Read the model definition and answer for the solid it produces. Units are mm, in the model's axes. A direction names the side the tool comes from. Give positions to 0.01 mm unless a question says otherwise; leave off trailing zeros. Write each loop counter-clockwise with the first axis right and the second up, starting at its lowest first coordinate (ties: lowest second). Pieces come first, ordered by that corner, then holes. Notation, with made-up numbers: (48, 84.5) - (75, 84.5) arc R15 ccw to (75, 101.5) - close; hole circle Ø4 at (61.25, 47). An arc over 180 degrees is marked (long way). Answer as CSV lines item,"result".
```python
from build123d import *

# Parameters (mm, degrees)
SKETCH2_R          = 2
CUT_EXTRUDE1_DEPTH = 10


with BuildPart() as part:
    # Sketch1 → Revolve1 (revolve)
    with BuildSketch(Plane.XY, mode=Mode.PRIVATE) as revolve1_sk:
        Polygon((0, 0), (132, 0), (132, 4), (114, 4), (114, 6), (112, 6), (112, 13), (110, 13), (110, 21), (0, 21), align=None)
    revolve(revolve1_sk.sketch.rotate(Axis((0, 0, 0), (1, 0, 0)), 180), axis=Axis((0, 0, 0), (1, 0, 0)))

    # Sketch2 → Cut-Extrude1 (cut)
    with BuildSketch(Plane(origin=(110, 0, 0), x_dir=(0, 0, -1), z_dir=(1, 0, 0))):
        with Locations(Location((0, 17.365813997, 0), (0, 0, 90))):
            Circle(SKETCH2_R)
        with Locations(Location((17.365813997, 0, 0), (0, 0, 90))):
            Circle(SKETCH2_R)
        with Locations(Location((0, -17.365813997, 0), (0, 0, 90))):
            Circle(SKETCH2_R)
        with Locations(Location((-17.365813997, 0, 0), (0, 0, 90))):
            Circle(SKETCH2_R)
    extrude(amount=-CUT_EXTRUDE1_DEPTH, mode=Mode.SUBTRACT)


solid = part.part
```
(1) Each of these flat-tipped pins is pushed along its axis until it touches: P1, Ø3, axis at x = 18, z = -11, coming from the +Y side; P2, Ø3, axis at y = 8, z = 11, coming from the +X side; P3, Ø1, axis at x = 61.5, y = 10, coming from the -Z side. Where does it stop, or does it pass through?
Worked out:
P1,"stops at y = 18.73"
P2,"stops at x = 112"
P3,"stops at z = -18.73"
(2) A cutting plane is placed at C-C (x = 30). Write down the section's boundary in (y, z), and give its area (3 significant figures).
Worked out:
outline,"circle Ø42 at (0, 0)"
area,"1,390 mm^2"
(3) A cutting plane is placed at A-A (z = 0). Write down the section's boundary in (x, y).
Worked out:
outline,"(0, -21) - (110, -21) - (110, -19.37) - (100, -19.37) - (100, -15.37) - (110, -15.37) - (110, -13) - (112, -13) - (112, -6) - (114, -6) - (114, -4) - (132, -4) - (132, 4) - (114, 4) - (114, 6) - (112, 6) - (112, 13) - (110, 13) - (110, 15.37) - (100, 15.37) - (100, 19.37) - (110, 19.37) - (110, 21) - (0, 21) - close"
(4) A cutting plane is placed at D-D (y = -18). Write down the section's boundary in (x, z), and give its area (3 significant figures).
Worked out:
outline,"(0, -10.82) - (110, -10.82) - (110, -1.9) - (100, -1.9) - (100, 1.9) - (110, 1.9) - (110, 10.82) - (0, 10.82) - close"
area,"2,340 mm^2"
(5) Find the intervals of material crossed by L1, parallel to Z at x = 103, y = 0; L2, parallel to Z at x = 108.5, y = 1.5; L3, parallel to X at y = 6, z = -5, in increasing order.
Worked out:
L1,"z = -21 to -19.37, -15.37 to 15.37, 19.37 to 21"
L2,"z = -20.95 to -18.69, -16.04 to 16.04, 18.69 to 20.95"
L3,"x = 0 to 112"
(6) For faces 1 (the flat face through (132, 0, 0)), 2 (the flat face through (100, -17, 0)), determine the directions among +Z, -Z, +X, -X, +Y, -Y from which every point of the face is accessible in a straight line to the end or side of a thin tool.
Worked out:
face 1,"+Z, -Z, +X, +Y, -Y"
face 2,"+X"
(7) The mould has two halves that part along Y. Classify faces 3 (the cylindrical face through (105.07, -0.43, -19.32)), 4 (the cylindrical face through (54.23, -20.03, -6.31)), 5 (the flat face through (110, 9, -10)): +Y half, -Y half, draft (parallel to the pull), parting line (faces both ways), or undercut.
Worked out:
face 3,"undercut"
face 4,"parting line"
face 5,"draft"
